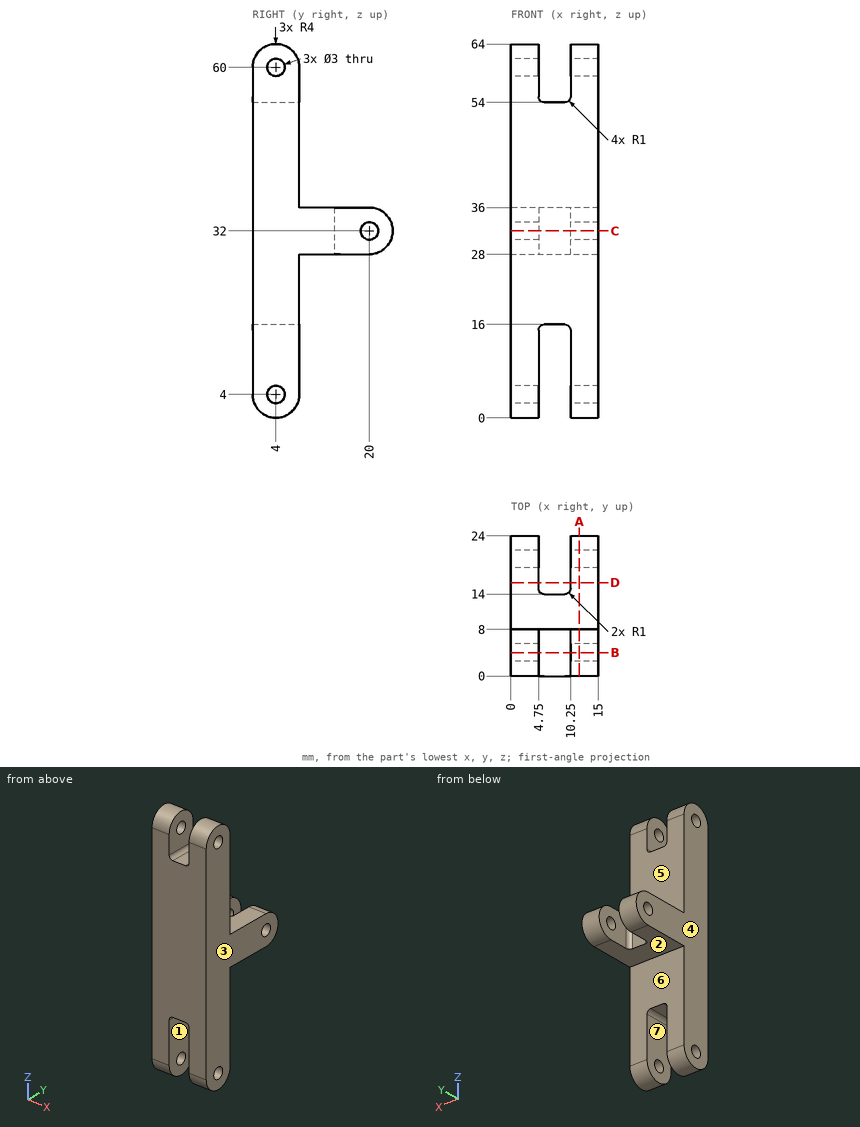
Design review of the part shown in the three views and the two pictorial views. Dimensions are in mm from the part's minimum x, y and z. A direction names the side the tool comes from. Coordinates: 2 decimals unless noted, no trailing zeros. Order: outer loops, then holes, each group sorted by start corner. A loop starts at its lowest first (then second) coordinate and runs counter-clockwise, first axis right, second up.
Item 1: Take a section at D-D, the plane y = 16. Write out the cut boundary in (x, z), then the cut area to 3 significant figures.
Item 2: For pin 1 Ø6 at (x, y) = (10.5, 13.5) entering from -Z; pin 2 Ø6 at (x, y) = (9, 13.5) entering from +Z; pin 3 Ø7.5 at (x, z) = (5.5, 21) entering from +Y, all flat-tipped, find the tip position at first contact; note any pin that passes through.
Item 3: For the marked faces 5, 6 and 7, list the 3-axis set-ups (+Z, -Z, +X, -X, +Y, -Y) from which the entire face can be reached by the end or side of a thin tool; tool diameter is ignored.
Item 4: Take a section at C-C, the plane z = 32. Write out the cut boundary in (x, y), then the cut area to 3 significant figures.
Item 5: Take a section at A-A, the plane x = 11.75. Write out the cut boundary in (y, z), then the cut area to 3 significant figures.
Item 6: Take a section at B-B, the plane y = 4. Count the separate pieces of the cut face and the enclosed holes in it, then the cut area to 3 significant figures.
Item 7: For line 1 (Z direction, x = 11.95, y = 4); line 2 (Y direction, x = 11.65, z = 60); line 3 (Y direction, x = 2.9, z = 32), list the stretches that pass through material, from the lowest coordinate up.
Item 8: The part is to be moulded in two halves that separate along X. For the marked faces 1, 2, 3 and 4, say which applies: pulls with the +X half, pulls with the -X half, needs draft (parallel to the pull), parting line crosses it, or undercut.
The answers:
1. outline: (0, 28) - (4.75, 28) - (4.75, 36) - (0, 36) - close; (10.25, 28) - (15, 28) - (15, 36) - (10.25, 36) - close
1. area: 76.0 mm2
2. pin 1: stops at z = 28
2. pin 2: stops at z = 36
2. pin 3: stops at y = 8
3. face 5: +Z, +X, -X, +Y
3. face 6: -Z, +X, -X, +Y
3. face 7: -Z, +Y, -Y
4. outline: (0, 0) - (15, 0) - (15, 18.5) - (10.25, 18.5) - (10.25, 15) arc R1 cw to (9.25, 14) - (5.75, 14) arc R1 cw to (4.75, 15) - (4.75, 18.5) - (0, 18.5) - close; (0, 21.5) - (4.75, 21.5) - (4.75, 24) - (0, 24) - close; (10.25, 21.5) - (15, 21.5) - (15, 24) - (10.25, 24) - close
4. area: 277 mm2
5. outline: (0, 4) arc R4 ccw to (8, 4) - (8, 28) - (20, 28) arc R4 ccw to (20, 36) - (8, 36) - (8, 60) arc R4 ccw to (0, 60) - close; hole circle Ø3 at (4, 4); hole circle Ø3 at (4, 60); hole circle Ø3 at (20, 32)
5. area: 598 mm2
6. separate pieces: 5
6. enclosed holes: 0
6. area: 761 mm2
7. line 1: z = 0 to 2.5, 5.5 to 58.5, 61.5 to 64
7. line 2: y = 0 to 2.5, 5.5 to 8
7. line 3: y = 0 to 18.5, 21.5 to 24
8. face 1: undercut
8. face 2: needs draft
8. face 3: pulls with the +X half
8. face 4: pulls with the -X half
